```python
from build123d import *

# Parameters (mm, degrees)
SKETCH_1_R          = 3.5
EXTRUDE_1_DEPTH     = 25
SKETCH_2_R          = 2
CUT_EXTRUDE_1_DEPTH = 20
SKETCH_3_R          = 2
CUT_EXTRUDE_2_DEPTH = 20


with BuildPart() as part:
    # 草图1 → 凸台-拉伸1 (new, symmetric)
    with BuildSketch(Plane.XY):
        Polygon((0, 0), (56.568542495, 56.568542495), (62.225396744, 50.911688245), (48.470353518, 37.156645019), (60.547431318, 8), (80, 8), (80, 0), align=None)
        with Locations((22.184677187, 9.156473773)):
            Circle(SKETCH_1_R, mode=Mode.SUBTRACT)
        Polygon((12.071067812, 5), (15.847671377, 8.776603565), (17.411991793, 5), align=None, mode=Mode.SUBTRACT)
        with BuildLine():
            Line((22.539170943, 15.468103131), (44.931612237, 37.860544425))
            Line((44.931612237, 37.860544425), (58.542895405, 5))
            Line((58.542895405, 5), (26.941798117, 5))
            ThreePointArc((26.941798117, 5), (26.493271042, 5.27903968), (26.545371373, 5.804706148))
            ThreePointArc((26.545371373, 5.804706148), (27.253512915, 11.291164467), (22.833720405, 14.61804341))
            ThreePointArc((22.833720405, 14.61804341), (22.420282519, 14.950846558), (22.539170943, 15.468103131))
        make_face(mode=Mode.SUBTRACT)
    extrude(amount=EXTRUDE_1_DEPTH, both=True)

    # 草图2 → 切除-拉伸1 (cut)
    with BuildSketch(Plane(origin=(0, 0, 0), x_dir=(0, 0, 1), z_dir=(-0.7071067811865488, 0.7071067811865464, 0))):
        with Locations(Location((-12.5, 70, 0), (0, 0, 270))):
            Circle(SKETCH_2_R)
        with Locations(Location((12.5, 70, 0), (0, 0, 270))):
            Circle(SKETCH_2_R)
    extrude(amount=-CUT_EXTRUDE_1_DEPTH, mode=Mode.SUBTRACT)

    # 草图3 → 切除-拉伸2 (cut)
    with BuildSketch(Plane.XZ):
        with Locations(Location((70, 12.5, 0), (0, 0, 270))):
            Circle(SKETCH_3_R)
        with Locations(Location((70, -12.5, 0), (0, 0, 270))):
            Circle(SKETCH_3_R)
    extrude(amount=-CUT_EXTRUDE_2_DEPTH, mode=Mode.SUBTRACT)


solid = part.part
```
Build history of the part. All positions in model axes, mm. A direction names the side the tool comes from. Give positions to 0.01 mm unless a question says otherwise; leave off trailing zeros. Loops run counter-clockwise (first coordinate to the right, second up) from the corner with the lowest first, then second, coordinate; pieces in that order, holes last. Notation, with made-up numbers: (86, 10) - (126, 10) arc R7 ccw to (126, 15) - close; hole circle Ø9 at (-6, 44.25). An arc over 180 degrees is marked (long way). Use a Markdown table: item, result.
(1) Wall check: line 1 along X through (y, z) = (7.5, 9); line 2 along X through (y, z) = (6, 5); line 3 along X through (y, z) = (6, 12.5). Give the ranges that are in metal, low to high.
Taken from the geometry:
| item | result |
|---|---|
| line 1 | 7.5 to 14.57, 16.38 to 19.1, 25.27 to 27.43, 57.51 to 80 |
| line 2 | 6 to 13.07, 17 to 20.67, 23.7 to 26.69, 58.13 to 80 |
| line 3 | 6 to 13.07, 17 to 20.67, 23.7 to 26.69, 58.13 to 68, 72 to 80 |
(2) Band-saw the part on B-B (x = 70). Give the cut face in (y, z).
Taken from the geometry:
| item | result |
|---|---|
| outline | (0, -25) - (8, -25) - (8, -14.5) - (0, -14.5) - close; (0, -10.5) - (8, -10.5) - (8, 10.5) - (0, 10.5) - close; (0, 14.5) - (8, 14.5) - (8, 25) - (0, 25) - close |
(3) Drop flat-ended pins along their axis: pin 1 Ø8 at (y, z) = (20, 5.5) entering from +X; pin 2 Ø6 at (x, z) = (15.5, -10.5) entering from +Y; pin 3 Ø4 at (x, z) = (39, 16.5) entering from +Y. Give the stop position or say it passes through.
Taken from the geometry:
| item | result |
|---|---|
| pin 1 | x = 57.23 |
| pin 2 | y = 18.5 |
| pin 3 | y = 41 |
(4) Pull direction Y, two halves, no side cores. Call faces 1 (the face through (41, 0, 0)), 2 (the face through (71.983, 3.944, -12.24)), 3 (the face through (54.424, 22.782, 0.35)): +Y half, -Y half, draft (parallel to the pull), parting line (faces both ways), or undercut.
Taken from the geometry:
| item | result |
|---|---|
| face 1 | -Y half |
| face 2 | draft |
| face 3 | undercut |
(5) Which spindle directions (+Z, -Z, +X, -X, +Y, -Y) get a long thin tool onto all of the face, cutting with end or side? Do faces 4 (the face through (55.444, 44.13, 0.35)), 5 (the face through (50.937, 45.36, 13.101)), 6 (the face through (16.62, 6.91, 0.35)). Say none if no direction does.
Taken from the geometry:
| item | result |
|---|---|
| face 4 | +Z, -Z, +X |
| face 5 | none |
| face 6 | +Z, -Z |
(6) Band-saw the part on D-D (y = 24.5). Give the cut face in (x, z).
Taken from the geometry:
| item | result |
|---|---|
| outline | (24.5, -25) - (31.57, -25) - (31.57, 25) - (24.5, 25) - close; (50.47, -25) - (53.71, -25) - (53.71, 25) - (50.47, 25) - close |
(7) Band-saw the part on C-C (x = 32). Give the cut face in (y, z).
Taken from the geometry:
| item | result |
|---|---|
| outline | (0, -25) - (5, -25) - (5, 25) - (0, 25) - close; (24.93, -25) - (32, -25) - (32, 25) - (24.93, 25) - close |
(8) Band-saw the part on A-A (z = -12.5). Give the cut face in (x, y).
Taken from the geometry:
| item | result |
|---|---|
| outline | (0, 0) - (68, 0) - (68, 8) - (60.55, 8) - (48.47, 37.16) - (53.74, 42.43) - (48.08, 48.08) - close; (50.91, 50.91) - (56.57, 45.25) - (62.23, 50.91) - (56.57, 56.57) - close; (72, 0) - (80, 0) - (80, 8) - (72, 8) - close; hole (12.07, 5) - (17.41, 5) - (15.85, 8.78) - close; hole circle Ø7 at (22.18, 9.16); hole (22.54, 15.47) arc R0.5 ccw to (22.83, 14.62) arc R5.5 cw to (26.55, 5.8) arc R0.5 ccw to (26.94, 5) - (58.54, 5) - (44.93, 37.86) - close |
